from build123d import *

# Parameters (mm, degrees)
F0_R     = 64.619688
F2_DEPTH = 74
F1_R     = 42.736697
F3_DEPTH = 74.001
F4_SIZE  = 20
F6_DEPTH = 102


with BuildPart() as f2:
    # F0 (on Top) → F2 (new body)
    with BuildSketch(Plane.XY):
        Circle(F0_R)
    extrude(amount=F2_DEPTH)

    # F1 (on Top) → F3 (cut, through all)
    with BuildSketch(Plane.XY):
        Circle(F1_R)
    extrude(amount=F3_DEPTH, mode=Mode.SUBTRACT)

    # F4
    f4_edges = [f2.edges().sort_by_distance(p)[0] for p in [
        (-64.619688, 0, 0),
    ]]
    chamfer(f4_edges, length=F4_SIZE)

    # F5 (on Top) → F6 (cut)
    with BuildSketch(Plane.XY):
        Polygon((-21.568869, -82.25935), (-0.245193, -97.784208), (21.109202, -82.301633), (12.983269, -57.208017), (-13.393229, -57.181884), align=None)
        Polygon((22.775318, -54.133459), (30.901251, -79.227075), (57.27775, -79.253207), (65.453389, -54.175742), (44.129714, -38.650883), align=None)
        Polygon((50.244468, -30.407892), (71.568144, -45.93275), (92.922539, -30.450175), (84.796606, -5.356559), (58.420108, -5.330426), align=None)
        Polygon((58.521939, 4.932456), (84.898438, 4.906324), (93.074077, 29.983789), (71.750402, 45.508648), (50.396006, 30.026072), align=None)
        Polygon((44.446018, 38.388774), (65.800414, 53.871349), (57.674481, 78.964965), (31.297982, 78.991097), (23.122343, 53.913632), align=None)
        Polygon((13.393229, 57.181884), (21.568869, 82.25935), (0.245193, 97.784208), (-21.109202, 82.301633), (-12.983269, 57.208017), align=None)
        Polygon((-22.775318, 54.133459), (-30.901251, 79.227075), (-57.27775, 79.253207), (-65.453389, 54.175742), (-44.129714, 38.650883), align=None)
        Polygon((-50.244468, 30.407892), (-71.568144, 45.93275), (-92.922539, 30.450175), (-84.796606, 5.356559), (-58.420108, 5.330426), align=None)
        Polygon((-58.521939, -4.932456), (-84.898438, -4.906324), (-93.074077, -29.983789), (-71.750402, -45.508648), (-50.396006, -30.026072), align=None)
        Polygon((-44.446018, -38.388774), (-65.800414, -53.871349), (-57.674481, -78.964965), (-31.297982, -78.991097), (-23.122343, -53.913632), align=None)
    extrude(amount=F6_DEPTH, mode=Mode.SUBTRACT)


solid = f2.part
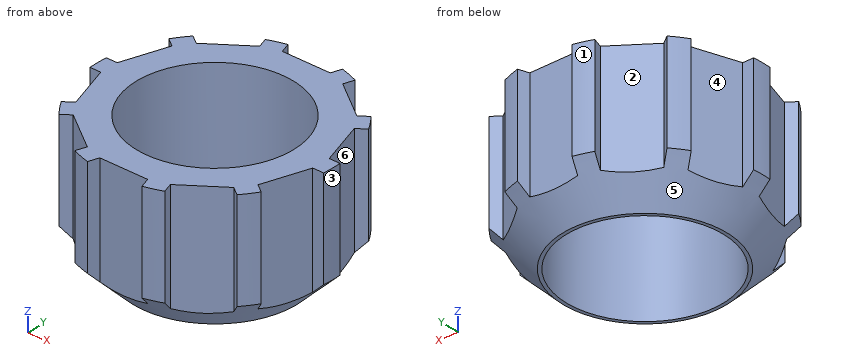
Verification items for the finished model (mm, model axes). Face numbers are marked on the shaded views. A direction names the side the tool comes from. Coordinates: 2 decimals unless noted, no trailing zeros. Order: outer loops, then holes, each group sorted by start corner. A loop starts at its lowest first (then second) coordinate and runs counter-clockwise, first axis right, second up. Notation, with made-up numbers: (44.25, 53) -> (72.25, 53) arc R15 cw to (72.25, 79) -> close; hole circle Ø5 at (35.25, 29). An arc over 180 degrees is marked (long way). Use CSV: the item, a comma, the result in double quotes. Start each with the question number.
Q1. Draft check along X on the marked faces 1, 2 and 3. Enter one of: +X half, -X half, draft (parallel to the pull), parting line (faces both ways), or undercut.
Q2. Section check A-A, the plane y = 0. Record the cut outline in (x, z), and give its area (3 significant figures).
Q3. Section check B-B, the plane x = 0. Record the cut outline in (y, z), and give its area (3 significant figures).
Q4. Section check C-C, the plane z = 10.5. Record the cut outline in (x, y), and give its area (3 significant figures).
Q5. Depth check by flat-ended pin: P1, Ø10, axis at y = -24, z = 35.5, coming from the +X side; P2, Ø1.5, axis at y = 41, z = 66, coming from the -X side; P3, Ø5, axis at x = -49, z = 51, coming from the -Y side. Enter the tip coordinate at first touch or a pass-through.
Q6. Thickness scan on line 1 along Y through (x, z) = (0, 33); line 2 along X through (y, z) = (0, 55); line 3 along Y through (x, z) = (-16.5, 38). Record the ranges inside material, lowest first.
Q7. Tool access check on the marked faces 4, 5 and 6. Record the directions out of +Z, -Z, +X, -X, +Y, -Y that give a thin tool (end or side, any length) a straight path to the whole face; none if there is none.
Returned:
1,face 1,"-X half"
1,face 2,"undercut"
1,face 3,"+X half"
2,outline,"(-64.62, 20) -> (-44.62, 0) -> (-42.74, 0) -> (-42.74, 74) -> (-64.62, 74) -> close; (42.74, 0) -> (44.62, 0) -> (64.62, 20) -> (64.62, 74) -> (42.74, 74) -> close"
2,area,"2,840 mm^2"
3,outline,"(-57.2, 12.58) -> (-44.62, 0) -> (-42.74, 0) -> (-42.74, 74) -> (-57.2, 74) -> close; (42.74, 0) -> (44.62, 0) -> (57.2, 12.58) -> (57.2, 74) -> (42.74, 74) -> close"
3,area,"1,980 mm^2"
4,outline,"circle Ø110.24 at (0, 0); hole circle Ø85.47 at (0, 0)"
4,area,"3,810 mm^2"
5,P1,"stops at x = 53.96"
5,P2,"stops at x = -50.55"
5,P3,"stops at y = -41.86"
6,line 1,"y = -57.2 to -42.74, 42.74 to 57.2"
6,line 2,"x = -64.62 to -42.74, 42.74 to 64.62"
6,line 3,"y = -62.48 to -39.42, 39.42 to 62.48"
7,face 4,"+Z, -Z, -X"
7,face 5,"-Z"
7,face 6,"+Z, -Z, +X"
